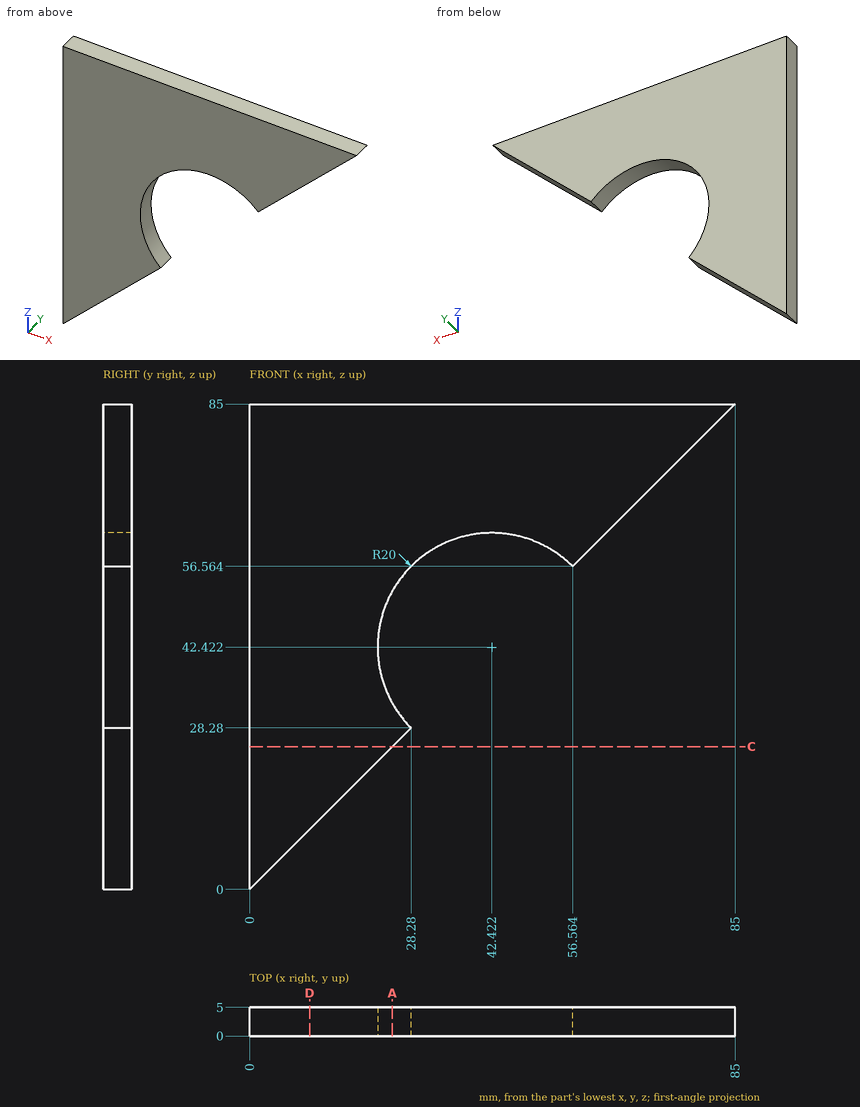
Part print with two shaded views. Sizes in mm from the minimum x, y, z corner. Round coordinates to 2 decimals unless told otherwise and drop trailing zeros. Order: outer loops, then holes, each group sorted by start corner. A loop starts at its lowest first (then second) coordinate and runs counter-clockwise, first axis right, second up. Notation, with made-up numbers: M 16,45 L 45,45 A17 cw 45,64 Z; hole C 5.25,12.25 d10. An arc over 180 degrees is marked long. Answer in a Markdown table with one row per item. Add a question column.
Q1. Wall check: L1, parallel to X at y = 2.4, z = 42; L2, parallel to Z at x = 28, y = 0.2 (1 decimal); L3, parallel to Z at x = 52.5, y = 1.45. Give the ranges that are in metal, low to high. Write a range as from..to.
Q2. Pin check, flat tips, straight feed: pin 1 (2 mm diameter, centred on x = 25, y = 1.5, fed in from -Z); pin 2 (3 mm diameter, centred on y = 4, z = 34.5, fed in from +X). Stop position of each tip, or through.
Q3. Cut at D-D on x = 10.5. Give the cut face in (y, z).
Q4. Cut at C-C on z = 25. Give the cut face in (x, y), and give its area (3 significant figures).
Q5. Cut at A-A on x = 25. Give the cut face in (y, z), and give its area (3 significant figures).
Established:
| question | item | result |
|---|---|---|
| 1 | L1 | x = 0..22.43 |
| 1 | L2 | z = 28..28.6, 56.3..85 |
| 1 | L3 | z = 59.7..85 |
| 2 | pin 1 | stops at z = 24 |
| 2 | pin 2 | stops at x = 24.78 |
| 3 | outline | M 0,10.5 L 5,10.5 L 5,85 L 0,85 Z |
| 4 | outline | M 0,0 L 25,0 L 25,5 L 0,5 Z |
| 4 | area | 125 mm2 |
| 5 | outline | M 0,25 L 5,25 L 5,32.6 L 0,32.6 Z; M 0,52.24 L 5,52.24 L 5,85 L 0,85 Z |
| 5 | area | 202 mm2 |
